```python
from build123d import *

# Parameters (mm, degrees)
ESBO_O1_W                = 54
ESBO_O1_H                = 54
RESSALTO_EXTRUS_O1_DEPTH = 180


with BuildPart() as part:
    # Esboço1 → Ressalto-extrusão1 (new, symmetric)
    with BuildSketch(Plane(origin=(0, 0, 0), x_dir=(1, 0, 0), z_dir=(0, 1, 0))):
        with BuildLine():
            Line((-28, -30), (28, -30))
            ThreePointArc((28, -30), (29.414213562, -29.414213562), (30, -28))
            Line((30, -28), (30, 28))
            ThreePointArc((30, 28), (29.414213562, 29.414213562), (28, 30))
            Line((28, 30), (-28, 30))
            ThreePointArc((-28, 30), (-29.414213562, 29.414213562), (-30, 28))
            Line((-30, 28), (-30, -28))
            ThreePointArc((-30, -28), (-29.414213562, -29.414213562), (-28, -30))
        make_face()
        Rectangle(ESBO_O1_W, ESBO_O1_H, mode=Mode.SUBTRACT)
    extrude(amount=RESSALTO_EXTRUS_O1_DEPTH, both=True)


solid = part.part
```
CAD build for the part. Positions are in the model's coordinates, mm. A direction names the side the tool comes from. Round coordinates to 2 decimals unless told otherwise and drop trailing zeros. Write each loop counter-clockwise with the first axis right and the second up, starting at its lowest first coordinate (ties: lowest second). Pieces come first, ordered by that corner, then holes. Notation, with made-up numbers: (24, 71) - (36, 71) arc R16 ccw to (36, 99) - close; hole circle Ø2 at (11, 51). An arc over 180 degrees is marked (long way). Return JSON: item names as keys, results as strings. Group by question number.
Item 1: Flat gauge pin, fed straight in: pin 1 Ø12 at (x, z) = (3.5, -16) entering from -Y. Where does the tip first touch, or does it go through?
Item 2: Band-saw the part on A-A on x = -3. List the corners of the cut face in (y, z), plus the area to 3 significant figures.
Item 3: Band-saw the part on C-C on y = 54. List the corners of the cut face in (x, z).
Item 4: Mould opens along Z. For faces 3 (the face through (-30, 3, 0)), 4 (the face through (-27, 3, 0)), 5 (the face through (0, 3, -30)) say: +Z half, -Z half, draft (parallel to the pull), parting line (faces both ways), or undercut.
Item 5: 3-axis set-ups, long thin cutter, end or side, ignore diameter. For faces 1 (the face through (0, 3, 30)), 2 (the face through (27, 3, 0)): which of +Z, -Z, +X, -X, +Y, -Y reach the whole face in a straight line?
Item 6: Probe probe 1 along X at (y, z) = (59.5, 12). List the from-to ranges inside material, lowest first.
Item 7: Band-saw the part on B-B on z = -13. List the corners of the cut face in (x, y).
Resolved:
{
 "1": {"pin 1": "passes through"},
 "2": {"outline": "(-180, -30) - (180, -30) - (180, -27) - (-180, -27) - close; (-180, 27) - (180, 27) - (180, 30) - (-180, 30) - close", "area": "2,160 mm²"},
 "3": {"outline": "(-30, -28) arc R2 ccw to (-28, -30) - (28, -30) arc R2 ccw to (30, -28) - (30, 28) arc R2 ccw to (28, 30) - (-28, 30) arc R2 ccw to (-30, 28) - close; hole (-27, -27) - (27, -27) - (27, 27) - (-27, 27) - close"},
 "4": {"face 3": "draft", "face 4": "undercut", "face 5": "-Z half"},
 "5": {"face 1": "+Z, +X, -X, +Y, -Y", "face 2": "+Y, -Y"},
 "6": {"probe 1": "x = -30 to -27, 27 to 30"},
 "7": {"outline": "(-30, -180) - (-27, -180) - (-27, 180) - (-30, 180) - close; (27, -180) - (30, -180) - (30, 180) - (27, 180) - close"}
}
